from build123d import *

# Parameters (mm, degrees)
F0_W     = 108.9
F0_H     = 76.3
F1_DEPTH = 15
F2_W     = 121.9
F2_H     = 87.3
F3_DEPTH = 15
F4_T     = -2.75
F7_DEPTH = 119


with BuildPart() as f1:
    # F0 (on Top) → F1 (new body)
    with BuildSketch(Plane.XY):
        Rectangle(F0_W, F0_H)
    extrude(amount=F1_DEPTH)

    # F2 (on Top) → F3 (join)
    with BuildSketch(Plane.XY):
        Rectangle(F2_W, F2_H)
    extrude(amount=F3_DEPTH)

    # F4
    f4_openings = [f1.faces().sort_by_distance(p)[0] for p in [
        (0, 0, 15),
    ]]
    offset(amount=F4_T, openings=f4_openings)

    # F6 (on face) → F7 (cut)
    with BuildSketch(Plane(origin=(60.95, 0, 0), x_dir=(0, -1, 0), z_dir=(-1, 0, 0))):
        Polygon((40.792018, 14.5), (40.792018, 15), (-40.792018, 15), (-40.792018, 14.5), (-41.829281, 13.878562), (-40.792018, 12.893027), (-40.792018, 12.20222), (40.792018, 12.20222), (40.792018, 12.893027), (41.829281, 13.878562), align=None)
    extrude(amount=F7_DEPTH, mode=Mode.SUBTRACT)


solid = f1.part
Read the model definition and answer for the solid it produces. Units are mm, in the model's axes. A direction names the side the tool comes from. Give positions to 0.01 mm unless a question says otherwise; leave off trailing zeros. Write each loop counter-clockwise with the first axis right and the second up, starting at its lowest first coordinate (ties: lowest second). Pieces come first, ordered by that corner, then holes. Notation, with made-up numbers: (-13.5, 81) -> (41.5, 81) arc R30 cw to (41.5, 103) -> close; hole circle Ø6 at (-4, 40.25). An arc over 180 degrees is marked (long way). Answer as a JSON object with one key per item and string values. Group by question number.
1) Consider L1, parallel to Y at x = -32, z = 12.5; L2, parallel to X at y = 14, z = 3.5; L3, parallel to Z at x = -53, y = 2.5. Determine where each line is inside the solid, lowest interval first. Write a range as from..to.
2) The mould has two halves that part along X. Classify faces 1 (the flat face through (-1, 1, 0)), 2 (the flat face through (-58.2, -1, 9)), 3 (the flat face through (60.95, -1, 6)): +X half, -X half, draft (parallel to the pull), parting line (faces both ways), or undercut.
3) A tool of negligible diameter and unlimited length cuts with its end or side. For faces 4 (the flat face through (58.2, -1, 7)), 5 (the flat face through (60, 1, 12.202)), 6 (the flat face through (-59, 0, 15)), from which of +Z, -Z, +X, -X, +Y, -Y can it reach the whole face along a straight path? Write none if from no direction.
4) Find section B-B (y = 30). Write down the section's boundary in (x, z), and give its area (3 significant figures).
5) Find section C-C (x = 27.5). Write down the section's boundary in (y, z).
6) Each of these flat-tipped pins is pushed along its axis until it touches: P1, Ø8, axis at x = -48.5, y = -4.5, coming from the +Z side; P2, Ø0.8, axis at x = 59, y = 15, coming from the +Z side. Where does it stop, or does it pass through?
7) Find section A-A (z = 6). Write down the section's boundary in (x, y), and give its area (3 significant figures).
Values follow:
{
 "1": {"L1": "y = -43.65..-40.9, 40.9..43.65", "L2": "x = -60.95..-58.2, 58.2..60.95", "L3": "z = 0..2.75"},
 "2": {"face 1": "draft", "face 2": "undercut", "face 3": "+X half"},
 "3": {"face 4": "+Z", "face 5": "+Z, +X", "face 6": "+Z, +X, -X, +Y, -Y"},
 "4": {"outline": "(-60.95, 0) -> (60.95, 0) -> (60.95, 12.2) -> (58.2, 12.2) -> (58.2, 2.75) -> (-58.2, 2.75) -> (-58.2, 15) -> (-60.95, 15) -> close", "area": "395 mm2"},
 "5": {"outline": "(-43.65, 0) -> (43.65, 0) -> (43.65, 15) -> (40.9, 15) -> (40.9, 14.44) -> (41.83, 13.88) -> (40.9, 13) -> (40.9, 2.75) -> (-40.9, 2.75) -> (-40.9, 13) -> (-41.83, 13.88) -> (-40.9, 14.44) -> (-40.9, 15) -> (-43.65, 15) -> close"},
 "6": {"P1": "stops at z = 2.75", "P2": "stops at z = 12.2"},
 "7": {"outline": "(-60.95, -43.65) -> (60.95, -43.65) -> (60.95, 43.65) -> (-60.95, 43.65) -> close; hole (-58.2, -40.9) -> (58.2, -40.9) -> (58.2, 40.9) -> (-58.2, 40.9) -> close", "area": "1,120 mm2"}
}
